Geometry: see drawing. Coordinates: mm, zero at the bounding-box minimum. A direction names the side the tool comes from. Coordinates: 2 decimals unless noted, no trailing zeros. Write each loop counter-clockwise with the first axis right and the second up, starting at its lowest first coordinate (ties: lowest second). Pieces come first, ordered by that corner, then holes. Notation, with made-up numbers: M 89.25,18 L 138.25,18 A32 cw 138.25,53 Z; hole C -31.75,-30.75 d8. An arc over 180 degrees is marked long. Write item = value, one per line. Start each with the question number.
1. Line query: line 1 along X through (y, z) = (3, 12); line 2 along Z through (x, y) = (10, 9.5); line 3 along Z through (x, y) = (11, 4.25). Output: solid intervals per line, ascending.
2. Pull-direction query (X, two-part tool) for the marked faces 1, 2, 3 and 4; classes: pulls with the +X half, pulls with the -X half, needs draft (parallel to the pull), parting line crosses it, or undercut.
3. Access query for the marked faces 5, 6 and 7. Directions: +Z, -Z, +X, -X, +Y, -Y. A direction counts if a zero-diameter tool reaches every point of the face in a straight line with its end or side. Return the directions, or none.
4. Pin query (flat end, axial travel): pin 1 Ø1.9 at (x, z) = (11.5, 40.5) entering from -Y; pin 2 Ø3 at (x, y) = (29.5, 4) entering from +Z; pin 3 Ø2 at (x, y) = (32, 4.5) entering from -Z. Return the tip coordinate at first contact, or that it passes through.
5. Section query C-C (y = 8). Output: boundary loops of the cut face in (x, z).
6. Section query B-B (z = 17.5). Output: boundary loops of the cut face in (x, y), then the cut area to 4 significant figures.
7. Section query D-D (y = 5.75). Output: boundary loops of the cut face in (x, z).
8. Section query A-A (x = 28). Output: boundary loops of the cut face in (y, z).
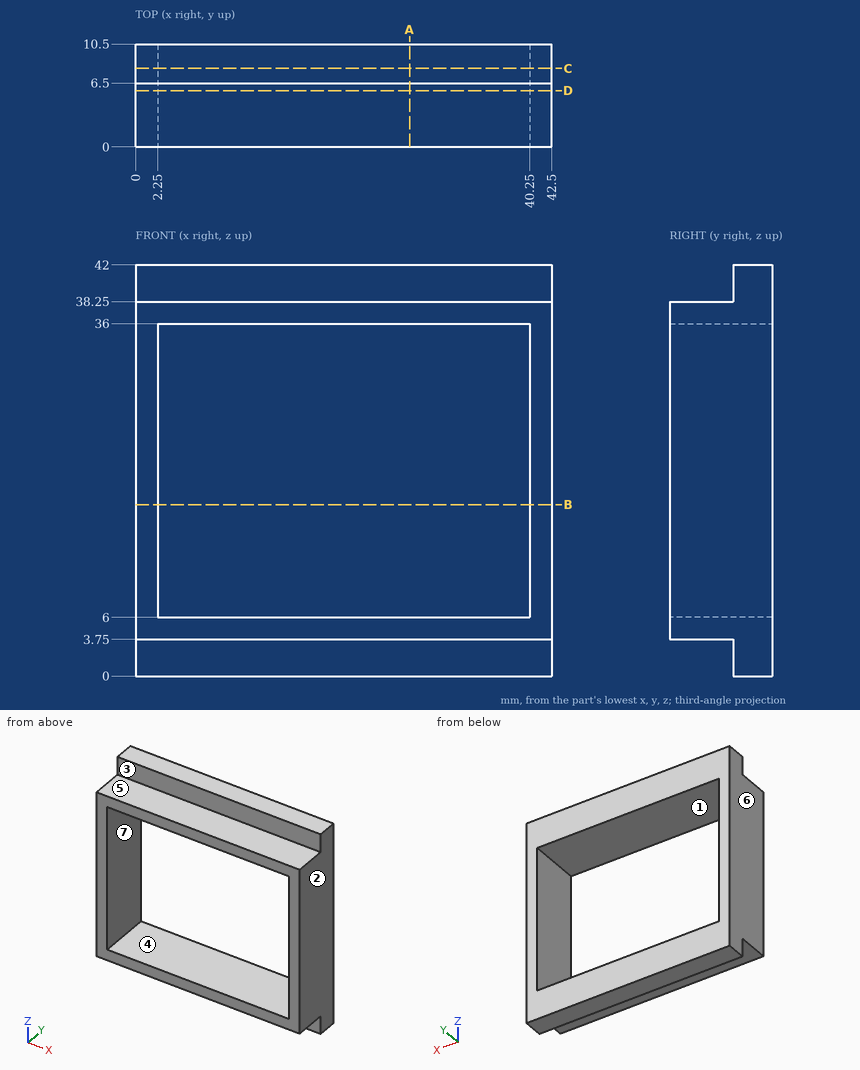
Results are:
q1.line_1 = 0 to 2.25, 40.25 to 42.5
q1.line_2 = 0 to 6, 36 to 42
q1.line_3 = 3.75 to 6, 36 to 38.25
q2.face_1 = undercut
q2.face_2 = pulls with the +X half
q2.face_3 = needs draft
q2.face_4 = undercut
q3.face_5 = +Z, +X, -X, -Y
q3.face_6 = +Z, -Z, -X, +Y, -Y
q3.face_7 = +Y, -Y
q4.pin_1 = 6.5
q4.pin_2 = 38.25
q4.pin_3 = 3.75
q5.outline = M 0,0 L 42.5,0 L 42.5,42 L 0,42 Z; hole M 2.25,6 L 40.25,6 L 40.25,36 L 2.25,36 Z
q6.outline = M 0,0 L 2.25,0 L 2.25,10.5 L 0,10.5 Z; M 40.25,0 L 42.5,0 L 42.5,10.5 L 40.25,10.5 Z
q6.area = 47.25 mm^2
q7.outline = M 0,3.75 L 42.5,3.75 L 42.5,38.25 L 0,38.25 Z; hole M 2.25,6 L 40.25,6 L 40.25,36 L 2.25,36 Z
q8.outline = M 0,3.75 L 6.5,3.75 L 6.5,0 L 10.5,0 L 10.5,6 L 0,6 Z; M 0,36 L 10.5,36 L 10.5,42 L 6.5,42 L 6.5,38.25 L 0,38.25 Z
